Build history of the part. All positions in model axes, mm. Face numbers are marked on the shaded views. A direction names the side the tool comes from. Round coordinates to 2 decimals unless told otherwise and drop trailing zeros. Write each loop counter-clockwise with the first axis right and the second up, starting at its lowest first coordinate (ties: lowest second). Pieces come first, ordered by that corner, then holes. Notation, with made-up numbers: (-30.5, 78.25) -> (2.5, 78.25) arc R21 cw to (2.5, 109.25) -> close; hole circle Ø5 at (87.25, 0.25). An arc over 180 degrees is marked (long way). One line per question, with ' | ' between items.
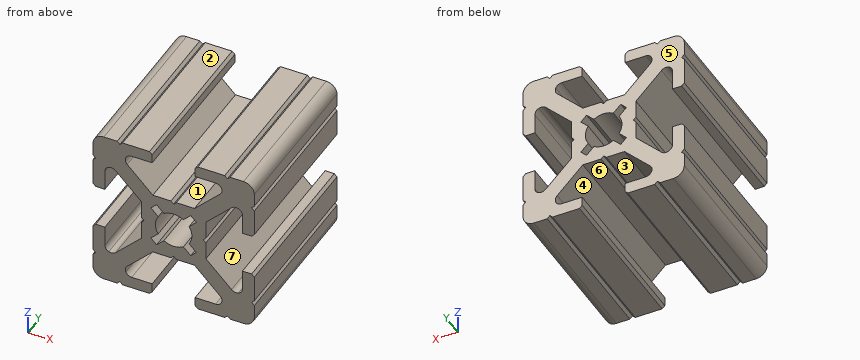
from build123d import *

# Parameters (mm, degrees)
F1_DEPTH = 30


# Not quite as in the source:
# - ends of sketch curves that miss each other by under 0.0002 mm in the source are joined


with BuildPart() as f1:
    # F0 (on Front) → F1 (new body)
    with BuildSketch(Plane.XZ):
        with BuildLine():
            ThreePointArc((-12.0672760652, 8.9096491574), (-11.3814883912, 8.9771930389), (-10.7737513132, 8.6523506868))
            Line((-10.7737513132, 8.6523506868), (-6, 3.8786))
            Line((-6, 3.8786), (-6, 0.5))
            Line((-6, 0.5), (-5.5, 0))
            Line((-5.5, 0), (-6, -0.5))
            Line((-6, -0.5), (-6, -3.8786))
            Line((-6, -3.8786), (-10.7738, -8.6524))
            ThreePointArc((-10.7738, -8.6524), (-11.3814883912, -8.9771930389), (-12.0672760652, -8.9096491574))
            ThreePointArc((-12.0672760652, -8.9096491574), (-12.5999492171, -8.4725051968), (-12.799999999, -7.8131))
            Line((-12.799999999, -7.8131), (-12.8, -4))
            Line((-12.8, -4), (-14.5, -4))
            Line((-14.5, -4), (-15, -4.5))
            Line((-15, -4.5), (-15, -9.5))
            Line((-15, -9.5), (-14.5, -10))
            Line((-14.5, -10), (-15, -10.5))
            Line((-15, -10.5), (-15, -13))
            ThreePointArc((-15, -13), (-14.4141844722, -14.4142216524), (-13, -15.0000239995))
            Line((-13, -15.0000239995), (-10.5, -15))
            Line((-10.5, -15), (-10, -14.5))
            Line((-10, -14.5), (-9.5, -15))
            Line((-9.5, -15), (-4.5, -15))
            Line((-4.5, -15), (-4, -14.5))
            Line((-4, -14.5), (-4, -12.8))
            Line((-4, -12.8), (-7.8131, -12.8))
            ThreePointArc((-7.8131, -12.8), (-8.4725048128, -12.5999494737), (-8.9096488038, -12.0672769187))
            ThreePointArc((-8.9096488038, -12.0672769187), (-8.977199798, -11.3815223738), (-8.6523996854, -10.7738003146))
            Line((-8.6523996854, -10.7738003146), (-3.8786, -6))
            Line((-3.8786, -6), (-0.5, -6))
            Line((-0.5, -6), (0, -5.5))
            Line((0, -5.5), (0.5, -6))
            Line((0.5, -6), (3.8786, -6))
            Line((3.8786, -6), (8.6524, -10.7738))
            ThreePointArc((8.6524, -10.7738), (8.977199798, -11.3815223738), (8.9096491574, -12.0672760652))
            ThreePointArc((8.9096491574, -12.0672760652), (8.4725048128, -12.5999494737), (7.8131, -12.799999999))
            Line((7.8131, -12.799999999), (4, -12.8))
            Line((4, -12.8), (4, -14.5))
            Line((4, -14.5), (4.5, -15))
            Line((4.5, -15), (9.5, -15))
            Line((9.5, -15), (10, -14.5))
            Line((10, -14.5), (10.5, -15))
            Line((10.5, -15), (13, -15))
            ThreePointArc((13, -15), (14.4141844722, -14.4142216524), (14.999955, -13.000024))
            Line((14.999955, -13.000024), (15, -10.5))
            Line((15, -10.5), (14.5, -10))
            Line((14.5, -10), (15, -9.5))
            Line((15, -9.5), (15, -4.5))
            Line((15, -4.5), (14.5, -4))
            Line((14.5, -4), (12.8, -4))
            Line((12.8, -4), (12.8, -7.8131))
            ThreePointArc((12.8, -7.8131), (12.5999492171, -8.4725051968), (12.0672760652, -8.9096491574))
            ThreePointArc((12.0672760652, -8.9096491574), (11.3814883912, -8.9771930389), (10.7737513132, -8.6523506868))
            Line((10.7737513132, -8.6523506868), (6, -3.8786))
            Line((6, -3.8786), (6, -0.5))
            Line((6, -0.5), (5.5, 0))
            Line((5.5, 0), (6, 0.5))
            Line((6, 0.5), (6, 3.8786))
            Line((6, 3.8786), (10.7738, 8.6524))
            ThreePointArc((10.7738, 8.6524), (11.3814883912, 8.9771930389), (12.0672760652, 8.9096491574))
            ThreePointArc((12.0672760652, 8.9096491574), (12.5999492171, 8.4725051968), (12.799999999, 7.8131))
            Line((12.799999999, 7.8131), (12.8, 4))
            Line((12.8, 4), (14.5, 4))
            Line((14.5, 4), (15, 4.5))
            Line((15, 4.5), (15, 9.5))
            Line((15, 9.5), (14.5, 10))
            Line((14.5, 10), (15, 10.5))
            Line((15, 10.5), (15, 13))
            ThreePointArc((15, 13), (14.4141844722, 14.4142216524), (13, 15.0000239995))
            Line((13, 15.0000239995), (10.5, 15))
            Line((10.5, 15), (10, 14.5))
            Line((10, 14.5), (9.5, 15))
            Line((9.5, 15), (4.5, 15))
            Line((4.5, 15), (4, 14.5))
            Line((4, 14.5), (4, 12.8))
            Line((4, 12.8), (7.8131, 12.8))
            ThreePointArc((7.8131, 12.8), (8.4725048128, 12.5999494737), (8.9096488038, 12.0672769187))
            ThreePointArc((8.9096488038, 12.0672769187), (8.977199798, 11.3815223738), (8.6523996854, 10.7738003146))
            Line((8.6523996854, 10.7738003146), (3.8786, 6))
            Line((3.8786, 6), (0.5, 6))
            Line((0.5, 6), (0, 5.5))
            Line((0, 5.5), (-0.5, 6))
            Line((-0.5, 6), (-3.8786, 6))
            Line((-3.8786, 6), (-8.6524, 10.7738))
            ThreePointArc((-8.6524, 10.7738), (-8.977199798, 11.3815223738), (-8.9096491574, 12.0672760652))
            ThreePointArc((-8.9096491574, 12.0672760652), (-8.4725048128, 12.5999494737), (-7.8131, 12.799999999))
            Line((-7.8131, 12.799999999), (-4, 12.8))
            Line((-4, 12.8), (-4, 14.5))
            Line((-4, 14.5), (-4.5, 15))
            Line((-4.5, 15), (-9.5, 15))
            Line((-9.5, 15), (-10, 14.5))
            Line((-10, 14.5), (-10.5, 15))
            Line((-10.5, 15), (-13, 15))
            ThreePointArc((-13, 15), (-14.4141844722, 14.4142216524), (-14.999955, 13.000024))
            Line((-14.999955, 13.000024), (-15, 10.5))
            Line((-15, 10.5), (-14.5, 10))
            Line((-14.5, 10), (-15, 9.5))
            Line((-15, 9.5), (-15, 4.5))
            Line((-15, 4.5), (-14.5, 4))
            Line((-14.5, 4), (-12.8, 4))
            Line((-12.8, 4), (-12.8, 7.8131))
            ThreePointArc((-12.8, 7.8131), (-12.5999492171, 8.4725051968), (-12.0672760652, 8.9096491574))
        make_face()
        with BuildLine():
            Line((-4.2426, -3.182), (-2.8752, -1.8146))
            ThreePointArc((-2.8752, -1.8146), (-3.4, 0), (-2.8752481958, 1.8146481236))
            Line((-2.8752481958, 1.8146481236), (-4.2426, 3.182))
            Line((-4.2426, 3.182), (-3.182, 4.2426))
            Line((-3.182, 4.2426), (-1.8146, 2.8752))
            ThreePointArc((-1.8146, 2.8752), (0, 3.4), (1.8146481236, 2.8752481958))
            Line((1.8146481236, 2.8752481958), (3.182, 4.2426))
            Line((3.182, 4.2426), (4.2426, 3.182))
            Line((4.2426, 3.182), (2.8752, 1.8146))
            ThreePointArc((2.8752, 1.8146), (3.4, 0), (2.8752481958, -1.8146481236))
            Line((2.8752481958, -1.8146481236), (4.2426, -3.182))
            Line((4.2426, -3.182), (3.182, -4.2426))
            Line((3.182, -4.2426), (1.8146, -2.8752))
            ThreePointArc((1.8146, -2.8752), (0, -3.4), (-1.8146481236, -2.8752481958))
            Line((-1.8146481236, -2.8752481958), (-3.182, -4.2426))
            Line((-3.182, -4.2426), (-4.2426, -3.182))
        make_face(mode=Mode.SUBTRACT)
    extrude(amount=F1_DEPTH)


solid = f1.part
(1) Slice it at B-B (z = 1). Write the cut outline in (x, y), then the cut area to 3 significant figures.
Calculated:
outline: (-6, -30) -> (-3.25, -30) -> (-3.25, 0) -> (-6, 0) -> close; (3.25, -30) -> (6, -30) -> (6, 0) -> (3.25, 0) -> close | area: 165 mm2
(2) 3-axis set-ups, long thin cutter, end or side, ignore diameter. For the marked faces 1, 2, 3 and 4: which of +Z, -Z, +X, -X, +Y, -Y reach the whole face in a straight line?
Calculated:
face 1: +Z, +Y, -Y | face 2: +Z, +X, -X, +Y, -Y | face 3: -Z, +Y, -Y | face 4: +Y, -Y
(3) Wall check: line 1 (X direction, y = -25.5, z = -8); line 2 (X direction, y = -10, z = 13); line 3 (X direction, y = -5.75, z = 7.5). Give the ranges that are in metal, low to high. Write a range as from..to.
Calculated:
line 1: -15..-12.79, -10.12..-5.88, 5.88..10.12, 12.79..15 | line 2: -15..-4, 4..15 | line 3: -15..-12.8, -9.62..-5.38, 5.38..9.62, 12.8..15
(4) Slice it at C-C (z = -5). Write the cut outline in (x, y).
Calculated:
outline: (-15, -30) -> (-12.8, -30) -> (-12.8, 0) -> (-15, 0) -> close; (-7.12, -30) -> (7.12, -30) -> (7.12, 0) -> (-7.12, 0) -> close; (12.8, -30) -> (15, -30) -> (15, 0) -> (12.8, 0) -> close
(5) Slice it at A-A (x = -11.5). Write the cut outline in (y, z), then the cut area to 3 significant figures.
Calculated:
outline: (-30, -15) -> (0, -15) -> (0, -8.99) -> (-30, -8.99) -> close; (-30, 8.99) -> (0, 8.99) -> (0, 15) -> (-30, 15) -> close | area: 360 mm2
(6) Drop flat-ended pins along their axis: pin 1 (4 mm diameter, centred on x = -1.5, y = -8, fed in from +Z); pin 2 (0.8 mm diameter, centred on y = -21, z = -13.5, fed in from +X); pin 3 (3.5 mm diameter, centred on y = -10.5, z = 2, fed in from +X). Give the stop position or say it passes through.
Calculated:
pin 1: z = 6 | pin 2: x = 15 | pin 3: x = 6
(7) Mould opens along Z. For the marked faces 5, 6 and 7 say: pulls with the +Z half, pulls with the -Z half, needs draft (parallel to the pull), parting line crosses it, or undercut.
Calculated:
face 5: needs draft | face 6: pulls with the -Z half | face 7: undercut
